```python
from build123d import *

# Parameters (mm, degrees)
SALIENTE_EXTRUIR1_DEPTH = 3
REDONDEO1_R             = 10
CROQUIS2_R              = 1.5
CROQUIS2_R_2            = 1.55
CORTAR_EXTRUIR1_DEPTH   = 135.610141171
CROQUIS4_W              = 110
CROQUIS4_H              = 50
CORTAR_EXTRUIR2_DEPTH   = 135.610141171
REDONDEO2_R             = 5
CROQUIS5_W              = 4
CROQUIS5_H              = 14.636342218
CORTAR_EXTRUIR3_DEPTH   = 135.610141171
CROQUIS6_W              = 14.636342218
CROQUIS6_H              = 3
SALIENTE_EXTRUIR2_DEPTH = 2
CROQUIS8_W              = 14.636342218
CROQUIS8_H              = 3
SALIENTE_EXTRUIR3_DEPTH = 2
CROQUIS9_R              = 2
CORTAR_EXTRUIR4_DEPTH   = 133.713564137


with BuildPart() as part:
    # Croquis1 → Saliente-Extruir1 (new body)
    with BuildSketch(Plane(origin=(0, 0, 0), x_dir=(1, 0, 0), z_dir=(0, 1, 0))):
        Polygon((-88.1, 42.318171109), (88.1, 42.318171109), (108.1, 22.318171109), (127.75, 22.318171109), (127.75, 7.681828891), (105.75, 7.681828891), (77.75, -42.318171109), (-77.75, -42.318171109), (-105.75, 7.681828891), (-127.75, 7.681828891), (-127.75, 22.318171109), (-108.1, 22.318171109), align=None)
    extrude(amount=SALIENTE_EXTRUIR1_DEPTH)

    # Redondeo1
    redondeo1_edges = [part.edges().sort_by_distance(p)[0] for p in [
        (-88.1, 1.5, -42.318171109),
        (88.1, 1.5, -42.318171109),
        (108.1, 1.5, -22.318171109),
        (105.75, 1.5, -7.681828891),
        (77.75, 1.5, 42.318171109),
        (-77.75, 1.5, 42.318171109),
        (-105.75, 1.5, -7.681828891),
        (-108.1, 1.5, -22.318171109),
    ]]
    fillet(redondeo1_edges, radius=REDONDEO1_R)

    # Croquis2 → Cortar-Extruir1 (cut, through all)
    with BuildSketch(Plane(origin=(0, 3, 0), x_dir=(1, 0, 0), z_dir=(0, 1, 0))):
        with Locations(Location((70, -27.318171109, 0), (0, 0, 270))):
            Circle(CROQUIS2_R)
        with Locations(Location((-70, -27.318171109, 0), (0, 0, 270))):
            Circle(CROQUIS2_R)
        with Locations(Location((-119.996067812, 15, 0), (0, 0, 270))):
            Circle(CROQUIS2_R_2)
        with Locations(Location((119.996067812, 15, 0), (0, 0, 270))):
            Circle(CROQUIS2_R_2)
        with Locations(Location((-17.5, -17.318171109, 0), (0, 0, 270))):
            Circle(CROQUIS2_R)
        with Locations(Location((17.5, -17.318171109, 0), (0, 0, 270))):
            Circle(CROQUIS2_R)
        with Locations(Location((-17.5, -37.318171109, 0), (0, 0, 270))):
            Circle(CROQUIS2_R)
        with Locations(Location((17.5, -37.318171109, 0), (0, 0, 270))):
            Circle(CROQUIS2_R)
    extrude(amount=-CORTAR_EXTRUIR1_DEPTH, mode=Mode.SUBTRACT)

    # Croquis4 → Cortar-Extruir2 (cut, through all)
    with BuildSketch(Plane(origin=(0, 3, 0), x_dir=(1, 0, 0), z_dir=(0, 1, 0))):
        with Locations((0, -17.318171109)):
            Rectangle(CROQUIS4_W, CROQUIS4_H)
    extrude(amount=-CORTAR_EXTRUIR2_DEPTH, mode=Mode.SUBTRACT)

    # Redondeo2
    redondeo2_edges = [part.edges().sort_by_distance(p)[0] for p in [
        (55, 1.5, 42.318171109),
        (-55, 1.5, 42.318171109),
        (-55, 1.5, -7.681828891),
        (55, 1.5, -7.681828891),
    ]]
    fillet(redondeo2_edges, radius=REDONDEO2_R)

    # Croquis5 → Cortar-Extruir3 (cut, through all)
    with BuildSketch(Plane(origin=(0, 3, 0), x_dir=(1, 0, 0), z_dir=(0, 1, 0))):
        with Locations((-125.75, 15)):
            Rectangle(CROQUIS5_W, CROQUIS5_H)
        with Locations((125.75, 15)):
            Rectangle(CROQUIS5_W, CROQUIS5_H)
    extrude(amount=-CORTAR_EXTRUIR3_DEPTH, mode=Mode.SUBTRACT)

    # Croquis6 → Saliente-Extruir2 (add)
    with BuildSketch(Plane(origin=(123.75, 0, 0), x_dir=(0, 0, -1), z_dir=(1, 0, 0))):
        with Locations((15, 1.5)):
            Rectangle(CROQUIS6_W, CROQUIS6_H)
    extrude(amount=SALIENTE_EXTRUIR2_DEPTH)

    # Croquis8 → Saliente-Extruir3 (add)
    with BuildSketch(Plane.ZY.offset(123.75)):
        with Locations((-15, 1.5)):
            Rectangle(CROQUIS8_W, CROQUIS8_H)
    extrude(amount=SALIENTE_EXTRUIR3_DEPTH)

    # Croquis9 → Cortar-Extruir4 (cut, through all)
    with BuildSketch(Plane(origin=(0, 3, 0), x_dir=(1, 0, 0), z_dir=(0, 1, 0))):
        with Locations(Location((-62.1, -35.218171109, 0), (0, 0, 270))):
            Circle(CROQUIS9_R)
    cortar_extruir4 = extrude(amount=-CORTAR_EXTRUIR4_DEPTH, mode=Mode.SUBTRACT)

    # Simetría1: Cortar-Extruir4 across plane
    add(cortar_extruir4.mirror(Plane(origin=(0, 0, 0), x_dir=(0, 0, 1), z_dir=(1, 0, 0))), mode=Mode.SUBTRACT)


solid = part.part
```
Input: part model. Units: mm. Frame: model coordinates. A direction names the side the tool comes from. Round coordinates to 2 decimals unless told otherwise and drop trailing zeros. Write each loop counter-clockwise with the first axis right and the second up, starting at its lowest first coordinate (ties: lowest second). Pieces come first, ordered by that corner, then holes. Notation, with made-up numbers: (71, 13.25) - (86, 13.25) arc R17 ccw to (86, 33.25) - close; hole circle Ø6 at (50, -11.5). An arc over 180 degrees is marked (long way). Write item = value, one per line.
(1) Pull-direction query (X, two-part tool) for faces 3 (the cylindrical face through (-63.874, 1.521, 36.141)), 4 (the flat face through (98, 1.48, -32.42)), 5 (the cylindrical face through (-76.881, 1.521, 40.983)); classes: +X half, -X half, draft (parallel to the pull), parting line (faces both ways), or undercut.
Geometry check:
face_3 = undercut
face_4 = +X half
face_5 = -X half
(2) Access query for faces 1 (the cylindrical face through (63.874, 1.521, 36.141)), 2 (the cylindrical face through (53.496, 1.479, -6.256)). Directions: +Z, -Z, +X, -X, +Y, -Y. A direction counts if a zero-diameter tool reaches every point of the face in a straight line with its end or side. Return the directions, or none.
Geometry check:
face_1 = +Y, -Y
face_2 = +Z, +Y, -Y
(3) Section query C-C on x = -87.5. Output: boundary loops of the cut face in (y, z).
Geometry check:
outline = (0, -41.67) - (3, -41.67) - (3, 24.91) - (0, 24.91) - close
(4) Material intervals for probe 1 along X at (y, z) = (0.7, -15); probe 2 along X at (y, z) = (1.45, -14); probe 3 along Z at (x, y) = (70, 1.5), sorted ascending.
Geometry check:
probe_1 = -125.75 to -121.55, -118.45 to 118.45, 121.55 to 125.75
probe_2 = -125.75 to -121.18, -118.81 to 118.81, 121.18 to 125.75
probe_3 = -42.32 to 25.82, 28.82 to 42.32
(5) Section query A-A on y = 0.85. State how many separate pieces and enclosed holes the cut face has, then the cut area to 3 significant figures.
Geometry check:
separate_pieces = 1
enclosed_holes = 6
area = 11,200 mm^2
(6) Contact query for flat-ended pins moving along their axis: pin 1 Ø4 at (x, z) = (70, 27.32) entering from -Y; pin 2 Ø1.5 at (y, z) = (1, 17) entering from -X; pin 3 Ø0.9 at (x, y) = (-116.5, 1) entering from +Z; pin 4 Ø0.9 at (y, z) = (1, 20.5) entering from +X. Output: stop coordinate, or through.
Geometry check:
pin_1 = 0
pin_2 = -92.35
pin_3 = -7.68
pin_4 = 90.22
(7) Section query B-B on z = -28. Output: boundary loops of the cut face in (x, y), then the cut area to 3 significant figures.
Geometry check:
outline = (-102.42, 0) - (102.42, 0) - (102.42, 3) - (-102.42, 3) - close
area = 615 mm^2
